Job drawing, mm, ordinate dimensions from the low corner. One solid piece. Coordinates: 2 decimals unless noted, no trailing zeros. Order: outer loops, then holes, each group sorted by start corner. A loop starts at its lowest first (then second) coordinate and runs counter-clockwise, first axis right, second up. Notation, with made-up numbers: (72, 19.5) - (108, 19.5) arc R12 ccw to (108, 23.5) - close; hole circle Ø3 at (-36.75, 74). An arc over 180 degrees is marked (long way). Use one line per item in the form item = value.
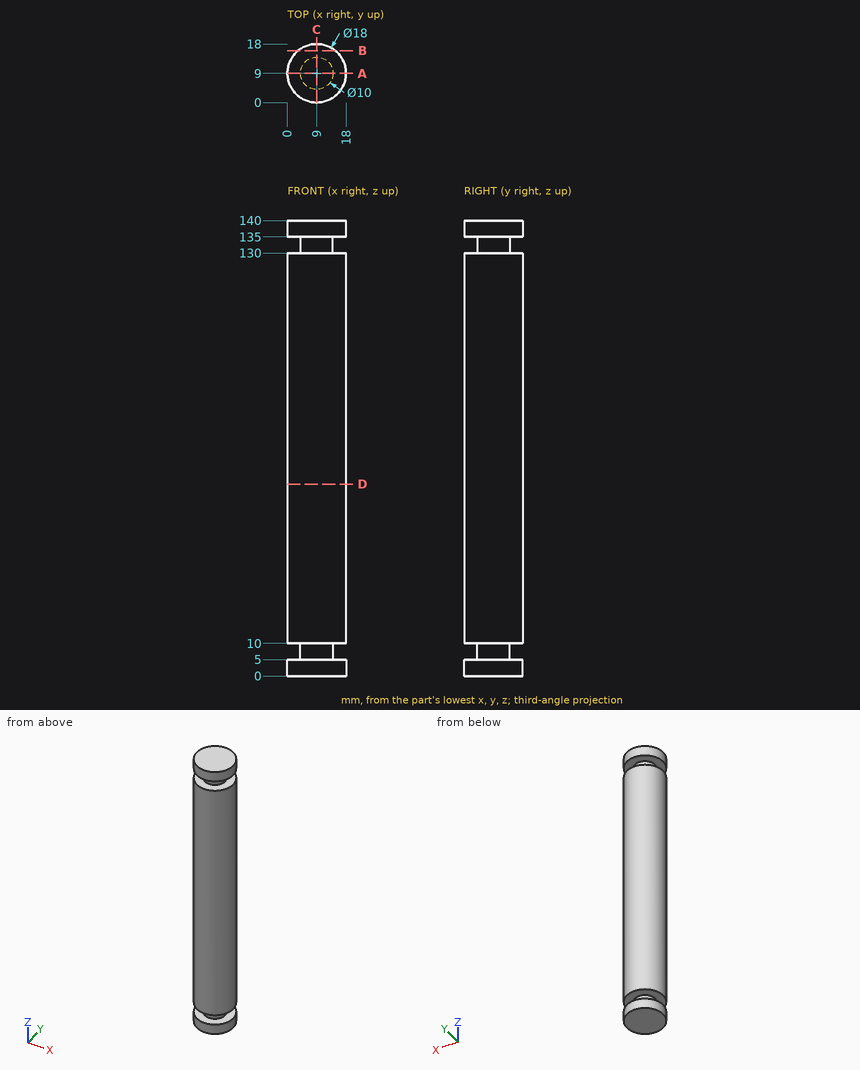
Item 1: Drill centre lines: line 1 (Z direction, x = 3, y = 4); line 2 (X direction, y = 8.5, z = 118); line 3 (X direction, y = 1.5, z = 56.5). Where is each one in solid material? Low to high. Write a range as [from, to].
Derived:
line_1 = [0, 5], [10, 130], [135, 140]
line_2 = [0.01, 17.99]
line_3 = [4.03, 13.97]
Item 2: Drop flat-ended pins along their axis: pin 1 (1.5 mm diameter, centred on y = 9.5, z = 36.5, fed in from +X); pin 2 (1 mm diameter, centred on x = 3.5, z = 84, fed in from +Y); pin 3 (4 mm diameter, centred on x = 5.5, z = 124, fed in from -Y); pin 4 (10 mm diameter, centred on y = 15.5, z = 122.5, fed in from +X). Give the stop position or say it passes through.
Derived:
pin_1 = 18
pin_2 = 16.48
pin_3 = 0.13
pin_4 = 17.87
Item 3: Cut at A-A, the plane y = 9. Write the cut outline in (x, z).
Derived:
outline = (0, 0) - (18, 0) - (18, 5) - (14, 5) - (14, 10) - (18, 10) - (18, 130) - (14, 130) - (14, 135) - (18, 135) - (18, 140) - (0, 140) - (0, 135) - (4, 135) - (4, 130) - (0, 130) - (0, 10) - (4, 10) - (4, 5) - (0, 5) - close
Item 4: Cut at D-D, the plane z = 59. Write the cut outline in (x, y).
Derived:
outline = circle Ø18 at (9, 9)
Item 5: Cut at B-B, the plane y = 16. Write the cut outline in (x, z).
Derived:
outline = (3.34, 0) - (14.66, 0) - (14.66, 5) - (3.34, 5) - close; (3.34, 10) - (14.66, 10) - (14.66, 130) - (3.34, 130) - close; (3.34, 135) - (14.66, 135) - (14.66, 140) - (3.34, 140) - close
